Geometry: final body of the model. Coordinates: model frame, mm. A direction names the side the tool comes from. Give positions to 0.01 mm unless a question says otherwise; leave off trailing zeros. Order: outer loops, then holes, each group sorted by start corner. A loop starts at its lowest first (then second) coordinate and runs counter-clockwise, first axis right, second up. Notation, with made-up numbers: (14.5, 40.25) -> (53.5, 40.25) arc R28 ccw to (53.5, 79.25) -> close; hole circle Ø11 at (12, -38.75). An arc over 180 degrees is marked (long way). Answer in a Markdown table with one row per item. Add a question column.
Q1. Cut plane A-A on y = 2.5. Return the cut outline in (x, z) (3 decimals), and give its area (3 significant figures).
Q2. Cut plane C-C on z = 33. Return the cut outline in (x, y) (3 decimals), and give its area (3 significant figures).
Q3. Contact query for a flat-ended pin moving along its axis: P1, Ø3, axis at x = -86.66, z = 68.19, coming from the -Y side. Output: stop coordinate, or through.
Q4. Cut plane D-D on x = -15.5. Return the cut outline in (y, z), and give its area (3 significant figures).
Q5. Pull-direction query (X, two-part tool) for faces 1 (the face through (3.556, 5, 36)), 2 (the face through (0, 3, 36)), 3 (the face through (-44, 5, -3.556)); classes: +X half, -X half, draft (parallel to the pull), parting line (faces both ways), or undercut.
Q6. Cut plane B-B on x = -50.5. Return the cut outline in (y, z).
Q7. Set-up query: faces 4 (the face through (-2.33, 8.12, 66.94)), 5 (the face through (-44, 3, 0)). Return all of +Z, -Z, +X, -X, +Y, -Y with unobstructed straight access to the full face (end or side cutting, diameter ignored); none if empty.
Q8. Line query: line 1 along X through (y, z) = (6, 38.5) (3 decimals); line 2 along Z through (x, y) = (-15, 5.5); line 3 along X through (y, z) = (9, 35.5) (3 decimals). Output: solid intervals per line, ascending. Write a range as from..to.
Autodesk Inventor part; units mm, degrees
ref_plane "YZ Plane" through (0, 0, 0) normal (1, 0, 0) x (0, 1, 0)
ref_plane "XZ Plane" through (0, 0, 0) normal (0, 1, 0) x (-1, 0, 0)
ref_plane "XY Plane" through (0, 0, 0) normal (0, 0, 1) x (1, 0, 0)
sketch "Sketch1" plane through (0, 0, 0) normal (0, 1, 0) x (-1, 0, 0)
  line L0 (0, 0) -> (89.789, 0)
  line L1 (89.789, 0) -> (89.789, 71.3232)
  line L2 (89.789, 71.3232) -> (0, 71.3232)
  line L3 (0, 71.3232) -> (0, 0)
  line L4 (93.345, 74.8792) -> (-3.556, 74.8792)
  line L5 (-3.556, 74.8792) -> (-3.556, -3.556)
  line L6 (-3.556, -3.556) -> (93.345, -3.556)
  line L7 (93.345, -3.556) -> (93.345, 74.8792)
  dimension "d0" = 89.789
  dimension "d1" = 71.3232
  dimension "d2" = 3.556
  dimension "d3" = 3.556
  dimension "d4" = 3.556
  dimension "d5" = 3.556
extrude "Extrusion1" add sketch "Sketch1" along normal blind 6.35
sketch "Sketch2" plane through (0, 6.35, 0) normal (0, 1, 0) x (1, 0, 0)
  line L0 (-93.345, 3.556) -> (3.556, 3.556)
  line L1 (3.556, 3.556) -> (3.556, -74.8792)
  line L2 (3.556, -74.8792) -> (-93.345, -74.8792)
  line L3 (-93.345, -74.8792) -> (-93.345, 3.556)
  point P0 (0, 0)
  dimension "d8" = 78.4352
  dimension "d9" = 96.901
extrude "Extrusion2" add sketch "Sketch2" along normal blind 3.556
sketch "Sketch3" plane through (0, 9.906, 0) normal (0, 1, 0) x (1, 0, 0)
  circle A0 centre (-44.8945, -35.6616) radius 8.0137
  line L0 (-93.345, 3.556) -> (-93.345, -74.8792)
  line L1 (3.556, 3.556) -> (-93.345, 3.556)
  point P0 (0, 0)
  dimension "d12" = 48.4505
  dimension "d13" = 39.2176
  dimension "d14" = 16.0274
extrude "Extrusion3" cut sketch "Sketch3" against normal blind 3.556 and the other way blind 1.016
sketch "Sketch5" plane through (-93.345, 0, -3.556) normal (-1, 0, 0) x (0, 0, 1)
  line L0 (78.4352, 0) -> (0, 0)
  line L1 (78.4352, 0) -> (77.1652, 0)
  line L2 (77.1652, 0) -> (77.1652, -7.62)
  line L3 (77.1652, -7.62) -> (78.4352, -7.62)
  line L4 (78.4352, -7.62) -> (78.4352, 0)
  line L5 (77.1652, -7.62) -> (76.4032, -6.5318)
  line L6 (76.4032, -6.5318) -> (76.4032, -2.54)
  line L7 (76.4032, -2.54) -> (77.1652, -2.54)
  point P0 (3.556, 0)
  dimension "d19" = 1.27
  dimension "d20" = 7.62
  dimension "d21" = 35
  dimension "d22" = 5.08
  dimension "d23" = 0.762
sketch "Sketch7" plane through (0, 9.906, 0) normal (0, 1, 0) x (1, 0, 0)
  circle A0 centre (-3.1305, -3.1305) radius 1.3525
  line L0 (0, 0) -> (0, -71.3232)
  line L1 (-89.789, 0) -> (0, 0)
  circle A1 centre (-3.1305, -3.1305) radius 3.1306
  dimension "d40" = 2.7051
  dimension "d41" = 6.2611
extrude "Extrusion6" cut sketch "Sketch7" along normal mid plane 25.4 contours A0
chamfer "Chamfer1" distance 1.905 angle 49 1 edges at (-4.4831, 9.906, 3.1305) measured on face at (-1.7824, 7.5353, 3.2394)
ref_plane "Work Plane4" through (-44.8945, 0, -3.556) normal (-1, 0, 0) x (0, 0, 1)
ref_plane "Work Plane5" through (3.556, 0, 35.6616) normal (0, 0, -1) x (-1, 0, 0)
mirror "Mirror3" about plane through (3.556, 0, 35.6616) normal (0, 0, -1) of "Extrusion6", "Chamfer1"
mirror "Mirror4" about plane through (-44.8945, 0, -3.556) normal (-1, 0, 0) of "Extrusion6", "Chamfer1", "Mirror3"
equation "\"d3\" = d2"
equation "\"d4\" = d2"
equation "\"d5\" = d2"
equation "\"d8\" = d1 + 2 * d3"
equation "\"d9\" = d0 + 2 * d3"
equation "\"d10\" = d3"
equation "\"d12\" = 0.5 * d9"
equation "\"d13\" = 0.5 * d8"
equation "\"d15\" = d3"
equation "\"d47\" = -d2 - 0.5 * d0"
equation "\"d48\" = -0.5 * d1 - d2"
properties part number "Masterboxtop"
Completed:
| question | item | result |
|---|---|---|
| 1 | outline | (-93.345, -3.556) -> (3.556, -3.556) -> (3.556, 74.879) -> (-93.345, 74.879) -> close; hole (-89.789, 0) -> (0, 0) -> (0, 71.323) -> (-89.789, 71.323) -> close |
| 1 | area | 1,200 mm² |
| 2 | outline | (-93.345, 0) -> (-89.789, 0) -> (-89.789, 6.35) -> (-52.453, 6.35) -> (-52.453, 9.906) -> (-93.345, 9.906) -> close; (-37.336, 6.35) -> (0, 6.35) -> (0, 0) -> (3.556, 0) -> (3.556, 9.906) -> (-37.336, 9.906) -> close |
| 2 | area | 336 mm² |
| 3 | P1 | stops at y = 6.35 |
| 4 | outline | (0, -3.56) -> (9.91, -3.56) -> (9.91, 74.88) -> (0, 74.88) -> (0, 71.32) -> (6.35, 71.32) -> (6.35, 0) -> (0, 0) -> close |
| 4 | area | 324 mm² |
| 5 | face 1 | +X half |
| 5 | face 2 | undercut |
| 5 | face 3 | draft |
| 6 | outline | (0, -3.56) -> (9.91, -3.56) -> (9.91, 29.93) -> (6.35, 29.93) -> (6.35, 0) -> (0, 0) -> close; (0, 71.32) -> (6.35, 71.32) -> (6.35, 41.39) -> (9.91, 41.39) -> (9.91, 74.88) -> (0, 74.88) -> close |
| 7 | face 4 | +Y |
| 7 | face 5 | -Y |
| 8 | line 1 | x = -93.345..-89.789, 0..3.556 |
| 8 | line 2 | z = -3.56..0, 71.32..74.88 |
| 8 | line 3 | x = -93.345..-52.907, -36.882..3.556 |
